Could you check a few things on this model? Use its own coordinates, in mm. Face numbers are marked on the shaded views. A direction names the side the tool comes from. Give positions to 0.01 mm unless a question says otherwise; leave off trailing zeros. Order: outer loops, then holes, each group sorted by start corner. A loop starts at its lowest first (then second) coordinate and runs counter-clockwise, first axis right, second up. Notation, with made-up numbers: (9, 13.5) - (15, 13.5) arc R21 ccw to (15, 30.5) - close; hole circle Ø7 at (-7.5, 48.25). An arc over 180 degrees is marked (long way). One line per question, with ' | ' between items. Start each with the question number.
1. Which directions (+Z, -Z, +X, -X, +Y, -Y) give clear straight access to the entire face, cutting with the end or side of a thin tool? Please do the marked faces 5, 6 and 7.
2. If we mould it in two halves opening along X, with no side actions, what happens to the marked faces 1, 2, 3 and 4? For each: released by +X, released by -X, zero draft, split by the parting line, or undercut.
3. Imagine slicing it at D-D (x = 55.5). Please give me the cut outline in (y, z) (3 decimals), and give its area (3 significant figures).
4. Imagine slicing it at C-C (x = 29). Please give me the cut outline in (y, z), and give its area (3 significant figures).
5. I need wall thicknesses on probe 1 along X at (y, z) = (17.5, 1); probe 2 along Z at (x, y) = (37, 0); probe 3 along Y at (x, z) = (31.5, 0.5). Which ranges of each line are inside material? Lowest first, please. Write a range as from..to.
6. Imagine slicing it at B-B (y = -7). Please give me the cut outline in (x, z) (3 decimals).
7. For P1, Ø6.5, axis at x = 59, y = -16.5, coming from the +Z side (3 decimals); P2, Ø16, axis at y = -13.5, z = -4, coming from the -X side; P3, Ø13, axis at x = 6.5, z = 33, coming from the -Y side; P4, Ø10, axis at x = 72, y = -14.5, coming from the +Z side, each with a flat end and sliding along its axis, tell me the tip position at first contact or that it passes through.
8. Imagine slicing it at A-A (y = 0). Please give me the cut outline in (x, z) (3 decimals), and give its area (3 significant figures).
```python
from build123d import *
from build123d import SkipClean  # not in build123d's __all__

# Parameters (mm, degrees)
F0_R           = 25.4
F0_R_2         = 12.7
F1_DEPTH       = 50.8
F3_DEPTH       = 38.1
F5_DEPTH       = 50.801
F6_DEPTH       = 25.4
F7_DEPTH       = 50.801
F9_DEPTH       = 25.4
F10_W          = 12.7
F10_H          = 34.925
F11_DEPTH      = 25.401
F11_DEPTH_BACK = 25.4


# Not quite as in the source:
# - a feature names something its author has since deleted; it is built from what else it names


with BuildPart() as f1:
    # F0 (on Right) → F1 (new body)
    with BuildSketch(Plane.YZ):
        Circle(F0_R)
        Circle(F0_R_2, mode=Mode.SUBTRACT)
    extrude(amount=F1_DEPTH)

    # F2 (on Right) → F3 (join)
    with BuildSketch(Plane.YZ):
        Polygon((-12.7, 38.1), (-12.7, 0), (25.4, 0), (25.4, 50.8), (12.7, 50.8), (12.7, 38.1), align=None)
    extrude(amount=F3_DEPTH)

    # F4 (on face) → F5 (cut, through all)
    with BuildSketch(Plane(origin=(0, 25.4, 0), x_dir=(-1, 0, 0), z_dir=(0, 1, 0))):
        Polygon((-38.1, 0), (0, 50.8), (-38.1, 50.8), align=None)
    extrude(amount=-F5_DEPTH, mode=Mode.SUBTRACT)

    # F6 (add): a face of the model
    f6_faces = [f1.faces().sort_by_distance(p)[0] for p in [
        (38.1, 19.05, 0.5679612663),
    ]]
    extrude(f6_faces, amount=F6_DEPTH)

    # F0 (on Right) → F7 (cut, through all)
    with BuildSketch(Plane.YZ):
        Circle(F0_R_2)
    extrude(amount=F7_DEPTH, mode=Mode.SUBTRACT)

    # F8 (on face) → F9 (join)
    with BuildSketch(Plane.YZ.offset(50.8)):
        with BuildLine():
            Line((-5.5358016583, 11.43), (-22.6829252964, 11.43))
            ThreePointArc((-22.6829252964, 11.43), (-5.8742530365, -24.7113971937), (25.4, 0))
            ThreePointArc((25.4, 0), (24.7113971937, 5.8742530365), (22.6829252964, 11.43))
            Line((22.6829252964, 11.43), (5.5358016583, 11.43))
            ThreePointArc((5.5358016583, 11.43), (10.7609172718, 6.7448246434), (12.7, 0))
            ThreePointArc((12.7, 0), (-6.7448246434, -10.7609172718), (-5.5358016583, 11.43))
        make_face()
    with SkipClean():  # cleaning this boolean's faces spoils the solid; the shape is the same uncleaned
        extrude(amount=F9_DEPTH)

    # F10 (on Front) → F11 (cut, two sides)
    with BuildSketch(Plane.XZ) as f11_sk:
        with Locations((57.15, 7.9375)):
            Rectangle(F10_W, F10_H)
    extrude(amount=-F11_DEPTH, mode=Mode.SUBTRACT)
    extrude(f11_sk.sketch, amount=F11_DEPTH_BACK, mode=Mode.SUBTRACT)


solid = f1.part
```
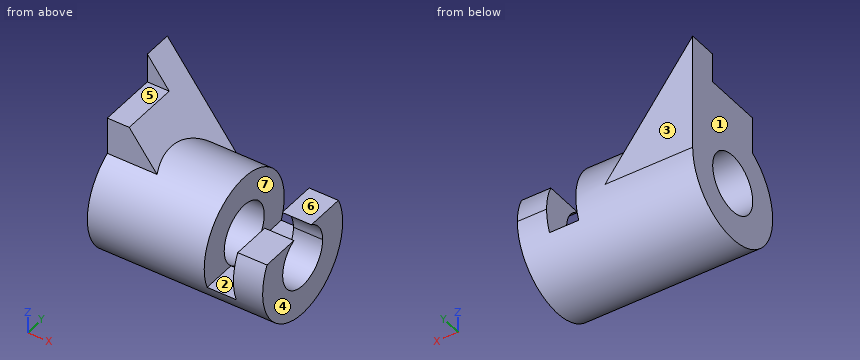
Results found:
1) face 5: +Z, +X, -X, -Y | face 6: +Z, +X, +Y, -Y | face 7: +Z, +Y, -Y
2) face 1: released by -X | face 2: undercut | face 3: zero draft | face 4: released by +X
3) outline: (-23.546, -9.525) arc R25.4 ccw to (23.546, -9.525) - (8.4, -9.525) arc R12.7 cw to (-8.4, -9.525) - close | area: 505 mm2
4) outline: (22.31, 12.13) arc R25.4 ccw (long way) to (25.4, 0) - (25.4, 12.13) - close; hole circle Ø25.4 at (0, 0) | area: 1,530 mm2
5) probe 1: x = 0..50.8, 63.5..76.2 | probe 2: z = -25.4..-12.7, 12.7..25.4 | probe 3: y = -25.4..-12.69, 12.69..25.4
6) outline: (0, -24.416) - (76.2, -24.416) - (76.2, -10.597) - (0, -10.597) - close; (0, 10.597) - (50.8, 10.597) - (50.8, 24.416) - (19.788, 24.416) - (9.525, 38.1) - (0, 38.1) - close; (63.5, 10.597) - (76.2, 10.597) - (76.2, 11.43) - (63.5, 11.43) - close
7) P1: stops at z = -9.525 | P2: stops at x = 0 | P3: stops at y = -12.7 | P4: stops at z = 11.43
8) outline: (0, -25.4) - (76.2, -25.4) - (76.2, -12.7) - (0, -12.7) - close; (0, 12.7) - (50.8, 12.7) - (50.8, 25.4) - (19.05, 25.4) - (9.525, 38.1) - (0, 38.1) - close | area: 1,790 mm2
